```python
from build123d import *

# Parameters (mm, degrees)
SKETCH1_W           = 106
SKETCH1_H           = 76
BOSS_EXTRUDE1_DEPTH = 60
BOSS_EXTRUDE2_DEPTH = 15
SKETCH3_R           = 14
BOSS_EXTRUDE3_DEPTH = 15
SKETCH4_R           = 5
BOSS_EXTRUDE4_DEPTH = 11
SKETCH5_R           = 11.5
BOSS_EXTRUDE5_DEPTH = 40
SKETCH6_R           = 8.5
BOSS_EXTRUDE6_DEPTH = 145


with BuildPart() as part:
    # Sketch1 → Boss-Extrude1 (new body)
    with BuildSketch(Plane(origin=(0, 0, 0), x_dir=(1, 0, 0), z_dir=(0, 1, 0))):
        Rectangle(SKETCH1_W, SKETCH1_H)
    extrude(amount=BOSS_EXTRUDE1_DEPTH)

    # Sketch2 → Boss-Extrude2 (add)
    with BuildSketch(Plane.XY.offset(38)):
        Polygon((9.237604307, 30), (4.618802154, 38), (-4.618802154, 38), (-9.237604307, 30), (-4.618802154, 22), (4.618802154, 22), align=None)
    extrude(amount=BOSS_EXTRUDE2_DEPTH)

    # Sketch3 → Boss-Extrude3 (add)
    with BuildSketch(Plane.XZ):
        Circle(SKETCH3_R)
    extrude(amount=BOSS_EXTRUDE3_DEPTH)

    # Sketch4 → Boss-Extrude4 (add)
    with BuildSketch(Plane.XZ.offset(15)):
        Circle(SKETCH4_R)
    extrude(amount=BOSS_EXTRUDE4_DEPTH)

    # Sketch5 → Boss-Extrude5 (add)
    with BuildSketch(Plane.XZ.offset(26)):
        Circle(SKETCH5_R)
    extrude(amount=BOSS_EXTRUDE5_DEPTH)

    # Sketch6 → Boss-Extrude6 (add)
    with BuildSketch(Plane.XZ.offset(66)):
        Circle(SKETCH6_R)
    extrude(amount=BOSS_EXTRUDE6_DEPTH)


solid = part.part
```
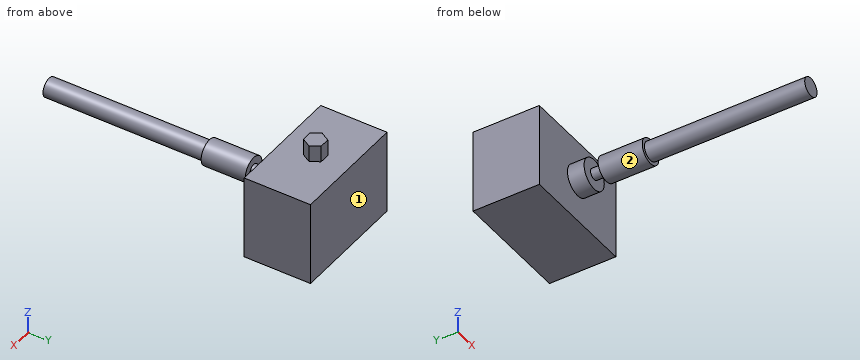
Check sheet for the modelled part. Datum: model origin and axes. Units: mm. Face numbers are marked on the shaded views. A direction names the side the tool comes from. Coordinates: 2 decimals unless noted, no trailing zeros. Order: outer loops, then holes, each group sorted by start corner. A loop starts at its lowest first (then second) coordinate and runs counter-clockwise, first axis right, second up. Notation, with made-up numbers: (-25.75, 82.5) -> (-5.75, 82.5) arc R24 cw to (-5.75, 116.5) -> close; hole circle Ø8 at (50, -0.5). An arc over 180 degrees is marked (long way). Write item = value, one per line. Start each with the question number.
1) Go/stop test with flat-tipped pins: P1, Ø10, axis at x = 0.5, y = -182, coming from the +Z side; P2, Ø8, axis at x = 6, z = -25.5, coming from the -Y side; P3, Ø5, axis at x = -7, y = 11, coming from the +Z side. Record where each tip stops, or that it passes through.
2) Access from +Z, -Z, +X, -X, +Y, -Y to the whole of each face (thin tool, end or side, straight path). Record for the marked faces 1 and 2.
3) Cross-section at A-A (x = 0). Enter the section's corners in (y, z).
4) Material ranges on L1, parallel to Y at x = -41, z = 37.5; L2, parallel to Y at x = 11.5, z = 2; L3, parallel to Z at x = 32, y = 15, recorded low to high.
5) Cross-section at B-B (z = 0). Enter the section's corners in (x, y).
6) Cross-section at C-C (y = -157.5). Enter the section's corners in (x, z).
7) Cross-section at D-D (z = 30). Enter the section's corners in (x, y), then the cut area to 3 significant figures.
Ans:
q1.P1 = 8.5
q1.P2 = 0
q1.P3 = 38
q2.face_1 = +Z, -Z, +X, -X, +Y
q2.face_2 = -Y
q3.outline = (-211, -8.5) -> (-66, -8.5) -> (-66, -11.5) -> (-26, -11.5) -> (-26, -5) -> (-15, -5) -> (-15, -14) -> (0, -14) -> (0, -38) -> (60, -38) -> (60, 38) -> (38, 38) -> (38, 53) -> (22, 53) -> (22, 38) -> (0, 38) -> (0, 14) -> (-15, 14) -> (-15, 5) -> (-26, 5) -> (-26, 11.5) -> (-66, 11.5) -> (-66, 8.5) -> (-211, 8.5) -> close
q4.L1 = 0 to 60
q4.L2 = -15 to 60
q4.L3 = -38 to 38
q5.outline = (-53, 0) -> (-14, 0) -> (-14, -15) -> (-5, -15) -> (-5, -26) -> (-11.5, -26) -> (-11.5, -66) -> (-8.5, -66) -> (-8.5, -211) -> (8.5, -211) -> (8.5, -66) -> (11.5, -66) -> (11.5, -26) -> (5, -26) -> (5, -15) -> (14, -15) -> (14, 0) -> (53, 0) -> (53, 60) -> (-53, 60) -> close
q6.outline = circle Ø17 at (0, 0)
q7.outline = (-53, 0) -> (53, 0) -> (53, 60) -> (-53, 60) -> close
q7.area = 6,360 mm²
